from build123d import *

# Parameters (mm, degrees)
F2_R = 2.54


with BuildPart() as f1:
    # F0 (on Front) → F1 (revolve)
    with BuildSketch(Plane.XZ):
        with BuildLine():
            ThreePointArc((-4.318, 28.2435778242), (-7.6873775939, 15.0668729236), (-14.2875, 3.175))
            Line((-14.2875, 3.175), (-14.2875, 0))
            Line((-14.2875, 0), (-7.3279, 0))
            Line((-7.3279, 0), (-7.3279, 9.906))
            Line((-7.3279, 9.906), (-3.556, 13.6779))
            Line((-3.556, 13.6779), (-3.556, 22.5698975516))
            ThreePointArc((-3.556, 22.5698975516), (-3.3626540126, 23.5419134698), (-2.8120512242, 24.3659487758))
            Line((-2.8120512242, 24.3659487758), (0, 27.178))
            Line((0, 27.178), (0, 46.228))
            add(Edge.make_bspline(
                [(0, 46.228), (-18.7837371747, 46.228), (-4.318, 28.2435778242)],
                knots=[0, 0, 0, 2.4498260338, 2.4498260338, 2.4498260338], degree=2, weights=[1, 0.3390278065, 1]))
        make_face()
    revolve(axis=Axis((0, 0, 36.703), (0, 0, -1)))

    # F2
    f2_edges = [f1.edges().sort_by_distance(p)[0] for p in [
        (4.318, 0, 28.243578),
        (14.2875, 0, 3.175),
    ]]
    fillet(f2_edges, radius=F2_R)


solid = f1.part
Design review of the part built by this model. Coordinates are the model's own, in mm. Round coordinates to 2 decimals unless told otherwise and drop trailing zeros. Write each loop counter-clockwise with the first axis right and the second up, starting at its lowest first coordinate (ties: lowest second). Pieces come first, ordered by that corner, then holes. Notation, with made-up numbers: (66.5, 50.25) - (119.5, 50.25) arc R14 cw to (119.5, 72.25) - close; hole circle Ø9 at (-15.5, 39). An arc over 180 degrees is marked (long way). Return JSON: item names as keys, results as strings. Group by question number.
Item 1: For probe 1 along Y at (x, z) = (0, 2.5); probe 2 along Y at (x, z) = (0, 5.5); probe 3 along X at (y, z) = (-2.75, 4.5), list the stretches that pass through material, from the lowest coordinate up. Write a range as [from, to].
Item 2: The part is to be moulded in two halves that separate along Y. For faces 1 (the face through (-13.2, -5.47, 1.16)), 2 (the face through (0.77, -3.47, 18.19)), 3 (the face through (7, 3, 0)), 4 (the face through (-3.57, 1.12, 13.49)), say which applies: pulls with the +Y half, pulls with the -Y half, needs draft (parallel to the pull), parting line crosses it, or undercut.
Item 3: We need section A-A on z = 7.5. Write out the cut boundary in (x, y).
Item 4: Insertion check: P1, Ø6, axis at y = 2.5, z = 33, coming from the -X side; P2, Ø8, axis at x = 0, y = 0, coming from the -Z side; P3, Ø11.5, axis at x = 0, y = 0, coming from the -Z side; P4, Ø6, axis at x = -9, y = 9.5, coming from the -Z side. Each pin has a flat end and moves straight along its axis. Give the tip position at first contact, or say it passes through.
Model answer:
{
 "1": {"probe 1": "y = [-14.28, -7.33], [7.33, 14.28]", "probe 2": "y = [-12.67, -7.33], [7.33, 12.67]", "probe 3": "x = [-13.06, -6.79], [6.79, 13.06]"},
 "2": {"face 1": "parting line crosses it", "face 2": "undercut", "face 3": "needs draft", "face 4": "undercut"},
 "3": {"outline": "circle Ø22.83 at (0, 0); hole circle Ø14.66 at (0, 0)"},
 "4": {"P1": "stops at x = -6.73", "P2": "stops at z = 13.23", "P3": "stops at z = 11.48", "P4": "stops at z = 0"}
}
